from build123d import *

# Parameters (mm, degrees)
SKETCH_W        = 20
SKETCH_H        = 32
PAD_DEPTH       = 6
SKETCH001_R     = 1.75
POCKET_DEPTH    = 6.001
SKETCH002_W     = 7
SKETCH002_H     = 18
POCKET001_DEPTH = 6.001
FILLET_R        = 3
SKETCH003_W     = 10
SKETCH003_H     = 3
PAD001_DEPTH    = 10
SKETCH004_R     = 3.25
POCKET002_DEPTH = 3.001
FILLET001_R     = 1


with BuildPart() as part:
    # Sketch → Pad (new body)
    with BuildSketch(Plane.XY):
        with Locations((10, 16)):
            Rectangle(SKETCH_W, SKETCH_H)
    extrude(amount=PAD_DEPTH)

    # Sketch001 (on Face6 of Pad) → Pocket (cut, through all)
    with BuildSketch(Plane.XY.offset(6)):
        with Locations((16, 28.5)):
            Circle(SKETCH001_R)
        with Locations((16, 3.5)):
            Circle(SKETCH001_R)
    extrude(amount=-POCKET_DEPTH, mode=Mode.SUBTRACT)

    # Sketch002 (on Face5 of Pocket) → Pocket001 (cut, through all)
    with BuildSketch(Plane.XY.offset(6)):
        with Locations((16.5, 16)):
            Rectangle(SKETCH002_W, SKETCH002_H)
    extrude(amount=-POCKET001_DEPTH, mode=Mode.SUBTRACT)

    # Fillet
    fillet_edges = [part.edges().sort_by_distance(p)[0] for p in [
        (20, 32, 3),
        (20, 25, 3),
        (20, 7, 3),
        (20, 0, 3),
    ]]
    fillet(fillet_edges, radius=FILLET_R)

    # Sketch003 (on Face5 of Fillet) → Pad001 (join)
    with BuildSketch(Plane.XY.offset(6)):
        with Locations((5, 30.5)):
            Rectangle(SKETCH003_W, SKETCH003_H)
    extrude(amount=PAD001_DEPTH)

    # Sketch004 (on Face18 of Pad001) → Pocket002 (cut, through all)
    with BuildSketch(Plane.XZ.offset(-29)):
        with Locations((5, 11)):
            Circle(SKETCH004_R)
    extrude(amount=-POCKET002_DEPTH, mode=Mode.SUBTRACT)

    # Fillet001
    fillet001_edges = [part.edges().sort_by_distance(p)[0] for p in [
        (5, 29, 6),
    ]]
    fillet(fillet001_edges, radius=FILLET001_R)


solid = part.part
Could you check a few things on this model? Use its own coordinates, in mm. A direction names the side the tool comes from. Coordinates: 2 decimals unless noted, no trailing zeros. Loops run counter-clockwise (first coordinate to the right, second up) from the corner with the lowest first, then second, coordinate; pieces in that order, holes last.
1. For faces 5 (the face through (19.1, 0.86, 3.04)), 6 (the face through (4.9, 29, 14.4)), 7 (the face through (15, 25, 3)), which set-ups out of +Z, -Z, +X, -X, +Y, -Y let a thin tool reach every point of the face, with its end or its side?
2. I need wall thicknesses on L1, parallel to Y at x = 16, z = 3.75; L2, parallel to Z at x = 5, y = 30.05; L3, parallel to Z at x = 12.5, y = 5.5. Which ranges of each line are inside material? Lowest first, please.
3. We'd pull the mould along X, two halves only. Please class faces 1 (the face through (6.75, 30.48, 13.74)), 2 (the face through (0, 19, 4)), 3 (the face through (10, 30, 11)), 4 (the face through (5, 31, 16)): released by +X, released by -X, zero draft, split by the parting line, or undercut.
4. Imagine slicing it at B-B (z = 11). Please give me the cut outline in (x, y).
5. Imagine slicing it at D-D (z = 4.25). Please give me the cut outline in (x, y).
6. Imagine slicing it at C-C (y = 3.5). Please give me the cut outline in (x, z), and give its area (3 significant figures).
7. For P1, Ø3, axis at x = 16, y = 28.5, coming from the +Z side; P2, Ø1.5, axis at y = 23.5, z = 2, coming from the +X side; P3, Ø4.5, axis at x = 16, y = 3.5, coming from the +Z side; P4, Ø7, axis at x = 6.5, z = 10.5, coming from the -Y side, each with a flat end and sliding along its axis, tell me the tip position at first contact or that it passes through.
8. Imagine slicing it at A-A (x = 5). Please give me the cut outline in (y, z).
Computed values:
1. face 5: +Z, -Z, +X, -Y
1. face 6: +Z, +X, -X, -Y
1. face 7: +Z, -Z, +X
2. L1: y = 0 to 1.75, 5.25 to 7, 25 to 26.75, 30.25 to 32
2. L2: z = 0 to 7.75, 14.25 to 16
2. L3: z = 0 to 6
3. face 1: undercut
3. face 2: released by -X
3. face 3: released by +X
3. face 4: zero draft
4. outline: (0, 29) - (1.75, 29) - (1.75, 32) - (0, 32) - close; (8.25, 29) - (10, 29) - (10, 32) - (8.25, 32) - close
5. outline: (0, 0) - (17, 0) arc R3 ccw to (20, 3) - (20, 4) arc R3 ccw to (17, 7) - (13, 7) - (13, 25) - (17, 25) arc R3 ccw to (20, 28) - (20, 29) arc R3 ccw to (17, 32) - (0, 32) - close; hole circle Ø3.5 at (16, 3.5); hole circle Ø3.5 at (16, 28.5)
6. outline: (0, 0) - (14.25, 0) - (14.25, 6) - (0, 6) - close; (17.75, 0) - (20, 0) - (20, 6) - (17.75, 6) - close
6. area: 99.0 mm2
7. P1: passes through
7. P2: stops at x = 13
7. P3: stops at z = 6
7. P4: stops at y = 29
8. outline: (0, 0) - (32, 0) - (32, 7.75) - (29, 7.75) - (29, 7) arc R1 cw to (28, 6) - (0, 6) - close; (29, 14.25) - (32, 14.25) - (32, 16) - (29, 16) - close
